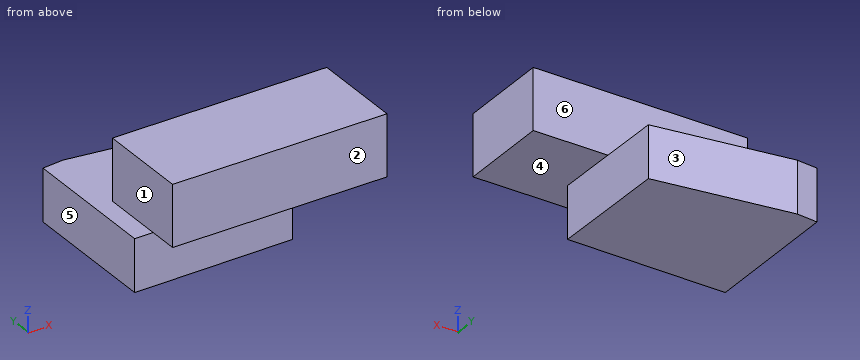
```python
from build123d import *

# Parameters (mm, degrees)
F1_DEPTH = 19.732377
F3_DEPTH = 23.135303


with BuildPart() as f1:
    # F0 (on Top) → F1 (new body)
    with BuildSketch(Plane.XY):
        Polygon((-16.213404, 28.059224), (-24.17749, 27.298637), (-24.17749, -25.769621), (35.927385, -25.125202), (35.433998, 20.8929), align=None)
    extrude(amount=F1_DEPTH)

    # F2 (on face) → F3 (join)
    with BuildSketch(Plane.XY.offset(19.732377)):
        Polygon((-17.158642, -2.116151), (-17.158642, -25.694368), (35.927385, -25.125202), (35.680692, -2.116151), align=None)
        Polygon((-17.158642, -25.694368), (-17.158642, -36.939867), (63.973717, -36.939867), (63.973717, -2.116151), (35.680692, -2.116151), (35.927385, -25.125202), align=None)
    extrude(amount=F3_DEPTH)


solid = f1.part
```
Check sheet for the modelled part. Datum: model origin and axes. Units: mm. Face numbers are marked on the shaded views. A direction names the side the tool comes from. Give positions to 0.01 mm unless a question says otherwise; leave off trailing zeros. Loops run counter-clockwise (first coordinate to the right, second up) from the corner with the lowest first, then second, coordinate; pieces in that order, holes last. Notation, with made-up numbers: (43, 5.5) - (73, 5.5) arc R31 ccw to (73, 35.5) - close; hole circle Ø8 at (33.25, 58). An arc over 180 degrees is marked (long way). One line per question, with ' | ' between items. Start each with the question number.
1. Draft check along X on the marked faces 1, 2 and 3. Enter one of: released by +X, released by -X, zero draft, split by the parting line, or undercut.
2. Material ranges on line 1 along Z through (x, y) = (53.5, -17); line 2 along Z through (x, y) = (-10, 3); line 3 along X through (y, z) = (-2, 10.5), recorded low to high. Write a range as [from, to].
3. Cross-section at A-A, the plane x = -11. Enter the section's corners in (y, z), plus the area to 3 significant figures.
4. Cross-section at D-D, the plane z = 30. Enter the section's corners in (x, y).
5. Cross-section at C-C, the plane z = 11.5. Enter the section's corners in (x, y).
6. Set-up check for the marked faces 4, 5 and 6: record each of +Z, -Z, +X, -X, +Y, -Y from which the full face is reachable in a straight line by a thin tool's end or side.
7. Gauge pin test, flat ends, axial feed: pin 1 Ø10.5 at (x, y) = (29.5, -20.5) entering from -Z; pin 2 Ø12 at (x, z) = (32.5, 25) entering from +Y; pin 3 Ø10 at (y, z) = (-23.5, 35) entering from -X; pin 4 Ø1.5 at (x, y) = (54.5, -3) entering from -Z. Record the tip position at first contact, or that the pin passes through.
8. Cross-section at B-B, the plane y = -8.5. Enter the section's corners in (x, z), plus the area to 3 significant figures.
Check result:
1) face 1: released by -X | face 2: zero draft | face 3: released by +X
2) line 1: z = [19.73, 42.87] | line 2: z = [0, 19.73] | line 3: x = [-24.18, 35.68]
3) outline: (-36.94, 19.73) - (-25.63, 19.73) - (-25.63, 0) - (27.34, 0) - (27.34, 19.73) - (-2.12, 19.73) - (-2.12, 42.87) - (-36.94, 42.87) - close | area: 1,850 mm2
4) outline: (-17.16, -36.94) - (63.97, -36.94) - (63.97, -2.12) - (-17.16, -2.12) - close
5) outline: (-24.18, -25.77) - (35.93, -25.13) - (35.43, 20.89) - (-16.21, 28.06) - (-24.18, 27.3) - close
6) face 4: -Z, +X, -Y | face 5: +Z, -Z, -X, +Y, -Y | face 6: +Z, +X, -X, +Y
7) pin 1: stops at z = 0 | pin 2: stops at y = 21.7 | pin 3: stops at x = -17.16 | pin 4: stops at z = 19.73
8) outline: (-24.18, 0) - (35.75, 0) - (35.75, 19.73) - (63.97, 19.73) - (63.97, 42.87) - (-17.16, 42.87) - (-17.16, 19.73) - (-24.18, 19.73) - close | area: 3,060 mm2
